Model file for the job. Use its own axes, mm. A direction names the side the tool comes from. Round coordinates to 2 decimals unless told otherwise and drop trailing zeros. Loops run counter-clockwise (first coordinate to the right, second up) from the corner with the lowest first, then second, coordinate; pieces in that order, holes last. Notation, with made-up numbers: (9, 45) - (35, 45) arc R26 ccw to (35, 82) - close; hole circle Ø4 at (85, 87.25). An arc over 180 degrees is marked (long way). Answer as a JSON object with one key per item and string values.
from build123d import *

# Parameters (mm, degrees)
PAD_DEPTH     = 75
SKETCH001_W   = 311.518585
SKETCH001_H   = 955.725281
PAD001_DEPTH  = 20
SKETCH002_W   = 275
SKETCH002_H   = 31.865801
PAD002_DEPTH  = 200
SKETCH003_W   = 1500
SKETCH003_H   = 970
PAD003_DEPTH  = 750
SKETCH004_W   = 890
SKETCH004_H   = 725
POCKET_DEPTH  = 750
SKETCH005_W   = 305
SKETCH005_H   = 245
SKETCH005_H_2 = 180
PAD004_DEPTH  = 25
SKETCH006_W   = 305
SKETCH006_H   = 185
SKETCH006_H_2 = 180
SKETCH006_W_2 = 890
SKETCH006_H_3 = 245
PAD005_DEPTH  = 25


with BuildPart() as part:
    # Sketch → Pad (new body)
    with BuildSketch(Plane.XZ):
        with BuildLine():
            Line((-750, -1000), (750, -1000))
            Line((750, -1000), (750, 1000))
            Line((750, 1000), (400, 1000))
            ThreePointArc((400, 1000), (0, 1400), (-400, 1000))
            Line((-400, 1000), (-750, 1000))
            Line((-750, 1000), (-750, -1000))
        make_face()
    extrude(amount=PAD_DEPTH)

    # Sketch001 (on Face8 of Pad) → Pad001 (join)
    with BuildSketch(Plane.XZ.offset(75)):
        with BuildLine():
            ThreePointArc((351.618271, 995.137056), (0, 1346.755326), (-351.618271, 995.137056))
            Line((-351.618271, 995.137056), (-351.618271, 0))
            Line((-351.618271, 0), (351.618271, 0))
            Line((351.618271, 995.137056), (351.618271, 0))
        make_face()
        with Locations((549.091598, 477.86264)):
            Rectangle(SKETCH001_W, SKETCH001_H)
        with Locations((-549.091598, 477.86264)):
            Rectangle(SKETCH001_W, SKETCH001_H)
    extrude(amount=PAD001_DEPTH)

    # Sketch002 (on Face21 of Pad001) → Pad002 (join)
    with BuildSketch(Plane.XZ.offset(95)):
        with Locations((-549.091599, 754.287087)):
            Rectangle(SKETCH002_W, SKETCH002_H)
        with Locations((-549.091599, 507.368162)):
            Rectangle(SKETCH002_W, SKETCH002_H)
        with Locations((-549.091599, 260.449237)):
            Rectangle(SKETCH002_W, SKETCH002_H)
        with Locations((549.091599, 754.287087)):
            Rectangle(SKETCH002_W, SKETCH002_H)
        with Locations((549.091599, 507.368162)):
            Rectangle(SKETCH002_W, SKETCH002_H)
        with Locations((549.091599, 260.449237)):
            Rectangle(SKETCH002_W, SKETCH002_H)
    extrude(amount=PAD002_DEPTH)

    # Sketch003 (on Face5 of Pad002) → Pad003 (join)
    with BuildSketch(Plane.XZ.offset(75)):
        with Locations((0, -515)):
            Rectangle(SKETCH003_W, SKETCH003_H)
    extrude(amount=PAD003_DEPTH)

    # Sketch004 (on Face12 of Pad003) → Pocket (cut)
    with BuildSketch(Plane.XZ.offset(825)):
        with Locations((0, -637.5)):
            Rectangle(SKETCH004_W, SKETCH004_H)
    extrude(amount=-POCKET_DEPTH, mode=Mode.SUBTRACT)

    # Sketch005 (on Face15 of Pocket) → Pad004 (join)
    with BuildSketch(Plane.XZ.offset(825)):
        with Locations((-597.5, -152.5)):
            Rectangle(SKETCH005_W, SKETCH005_H)
        with Locations((-597.5, -550)):
            Rectangle(SKETCH005_W, SKETCH005_H_2)
        with Locations((-597.5, -910)):
            Rectangle(SKETCH005_W, SKETCH005_H_2)
        with Locations((597.5, -152.5)):
            Rectangle(SKETCH005_W, SKETCH005_H)
        with Locations((597.5, -550)):
            Rectangle(SKETCH005_W, SKETCH005_H_2)
        with Locations((597.5, -910)):
            Rectangle(SKETCH005_W, SKETCH005_H_2)
    extrude(amount=-PAD004_DEPTH)

    # Sketch006 (on Face35 of Pad004) → Pad005 (join)
    with BuildSketch(Plane.XZ.offset(825)):
        with Locations((-597.5, -367.5)):
            Rectangle(SKETCH006_W, SKETCH006_H)
        with Locations((-597.5, -730)):
            Rectangle(SKETCH006_W, SKETCH006_H_2)
        with Locations((597.5, -367.5)):
            Rectangle(SKETCH006_W, SKETCH006_H)
        with Locations((597.5, -730)):
            Rectangle(SKETCH006_W, SKETCH006_H_2)
        with Locations((0, -152.5)):
            Rectangle(SKETCH006_W_2, SKETCH006_H_3)
    extrude(amount=-PAD005_DEPTH)


with BuildPart() as part_1:
    # Body placement: moved
    add(part.part.moved(Location((0, 412.5, 0))))


solid = part_1.part
1) Slice it at A-A on y = 198. Count the separate pieces of the cut face and the enclosed holes in it, then the cut area to 3 significant figures.
Values follow:
{"separate pieces": "7", "enclosed holes": "0", "area": "862,000 mm²"}
2) Probe probe 1 along Z at (x, y) = (-579.5, 157.5); probe 2 along X at (y, z) = (-340.5, -640); probe 3 along Y at (x, z) = (-389.5, 405). List the from-to ranges inside material, lowest first.
Values follow:
{"probe 1": "-1000 to -30, 244.52 to 276.38, 491.44 to 523.3, 738.35 to 770.22", "probe 2": "-750 to -445, 445 to 750", "probe 3": "337.5 to 412.5"}
3) Tool access for faces 1 (the cylindrical face through (7.73, 327.64, 1346.67)), 2 (the flat face through (-6, -43, -275)), 3 (the flat face through (547, 219, 770.22)), 4 (the flat face through (-551, 219, 276.382)): list every direction of +Z, -Z, +X, -X, +Y, -Y with a clear straight run to the whole face (end or side of a thin tool).
Values follow:
{"face 1": "+Z, -Y", "face 2": "-Z, -Y", "face 3": "+Z, +X, -X, -Y", "face 4": "+X, -X, -Y"}
4) Slice it at C-C on z = -312. List the corners of the cut face in (x, y).
Values follow:
{"outline": "(-750, -412.5) - (-445, -412.5) - (-445, 337.5) - (445, 337.5) - (445, -412.5) - (750, -412.5) - (750, 412.5) - (-750, 412.5) - close"}
5) Slice it at B-B on x = 0. List the corners of the cut face in (y, z), then the cut area to 3 significant figures.
Values follow:
{"outline": "(-412.5, -275) - (337.5, -275) - (337.5, -1000) - (412.5, -1000) - (412.5, 1400) - (337.5, 1400) - (337.5, 1346.76) - (317.5, 1346.76) - (317.5, 0) - (337.5, 0) - (337.5, -30) - (-412.5, -30) - close", "area": "391,000 mm²"}
6) Slice it at D-D on y = -188. List the corners of the cut face in (x, z), then the cut area to 3 significant figures.
Values follow:
{"outline": "(-750, -1000) - (-445, -1000) - (-445, -275) - (445, -275) - (445, -1000) - (750, -1000) - (750, -30) - (-750, -30) - close", "area": "810,000 mm²"}
7) Drop flat-ended pins along their axis: P1, Ø10, axis at y = 325, z = 305.5, coming from the -X side; P2, Ø10, axis at x = -89.5, y = 257.5, coming from the -Z side; P3, Ø16, axis at y = 186, z = 267.5, coming from the -X side; P4, Ø22, axis at x = 149, y = 328.5, coming from the -Z side. Give the stop position or say it passes through.
Values follow:
{"P1": "x = -704.85", "P2": "z = -275", "P3": "x = -686.59", "P4": "z = -1000"}
